Autodesk Fusion 360 part; units mm, degrees
sphere "SpherePrimitive2" add diameter 17 placed x (1, 0, 0) y (0, 0, -1) z (0, 1, 0) at (0, 0, 0) makes body 1
shell "Shell1" thickness 1 removed faces 0 bodies 1
ref_plane "WorkPlane1" through (0, 0, 3) normal (0, 0, 1) x (1, 0, 0)
split "Split1" by plane through (0, 0, 3) normal (0, 0, 1) bodies 1 makes body 2 at (-5.4981, 0.571, 6.4572)
delete_body "RemoveBody1" bodies 2
cylinder "CylinderPrimitive1" add diameter 17 height -22.5 placed x (1, 0, 0) y (0, 1, 0) z (0, 0, 1) at (0, 0, 0) separate body makes body 3
sphere "SpherePrimitive4" cut diameter 15 placed x (1, 0, 0) y (0, 0, -1) z (0, 1, 0) at (0, 0, 0) bodies 3
combine "Combine8" operation add target body 1 tool bodies 3
ref_plane "WorkPlane4" through (0, 8.5, -11.25) normal (0, 1, 0) x (1, 0, 0)
sketch "Sketch vis haut" plane through (0, 8.5, -4.25) normal (0, 1, 0) x (1, 0, 0)
  line L0 (0, 18.25) -> (0, 16.75)
  line L1 (-3, 18.25) -> (3, 18.25)
  line L2 (3, 18.25) -> (3, 15.25)
  line L3 (3, 15.25) -> (-3, 15.25)
  line L4 (-3, 15.25) -> (-3, 18.25)
  line L5 (0, 16.75) -> (0.1, 16.75)
  point P0 (0, 16.75)
  point P1 (0, 18.25)
  dimension "d72" = 1.5
  dimension "d73" = 3
  dimension "d74" = 6
extrude "Extrude4" add sketch "Sketch vis haut" along normal blind 6 and the other way blind 2 separate body makes body 4
hole "Hole1" at (0, 12.5, -19.5) direction (0, 0, -1) diameter 3 depth 3 tip angle 180 bodies 4
mirror "Mirror4" about plane through (0, 0, 0) normal (0, 1, 0) of bodies 4 makes body 5
combine "Combine9" operation add target body 1 tool bodies 4 5
sketch "Sketch13" plane through (0, 0, 3) normal (0, 0, 1) x (1, 0, 0)
  line L0 (9, 3.5) -> (-9, 3.5)
  line L1 (-9, 3.5) -> (-9, -3.5)
  line L2 (-9, -3.5) -> (9, -3.5)
  line L3 (9, -3.5) -> (9, 3.5)
  line L4 (9, 3.5) -> (-9, -3.5) construction
  line L5 (-9, 3.5) -> (9, -3.5) construction
  dimension "d54" = 7
  dimension "d55" = 18
extrude "Extrude5" cut sketch "Sketch13" against normal blind 10 bodies 1
Build history of the part. All positions in model axes, mm. A direction names the side the tool comes from. Give positions to 0.01 mm unless a question says otherwise; leave off trailing zeros. Loops run counter-clockwise (first coordinate to the right, second up) from the corner with the lowest first, then second, coordinate; pieces in that order, holes last. Notation, with made-up numbers: (-11, -40) -> (-2, -40) arc R17 cw to (-2, -14) -> close; hole circle Ø10 at (48, -8.5). An arc over 180 degrees is marked (long way). Answer in a Markdown table with one row per item.
Item 1: Tool access for faces 1 (the flat face through (-2, 2.4, -7)), 2 (the flat face through (-3, 11, -21)), 3 (the cylindrical face through (-8.49, 0.37, -11.09)), 4 (the flat face through (-3, -11, -21)), 5 (the flat face through (3, -11, -21)): list every direction of +Z, -Z, +X, -X, +Y, -Y with a clear straight run to the whole face (end or side of a thin tool).
Findings below:
| item | result |
|---|---|
| face 1 | +Z, +X, -X |
| face 2 | +Z, -Z, -X, +Y |
| face 3 | +Z |
| face 4 | +Z, -Z, -X, -Y |
| face 5 | +Z, -Z, +X, -Y |
Item 2: Slice it at A-A on y = -12.5. Write the cut outline in (x, z).
Findings below:
| item | result |
|---|---|
| outline | (-3, -22.5) -> (-1.5, -22.5) -> (-1.5, -19.5) -> (-3, -19.5) -> close; (1.5, -22.5) -> (3, -22.5) -> (3, -19.5) -> (1.5, -19.5) -> close |
Item 3: Slice it at D-D on y = 0. Write the cut outline in (x, z), plus the area to 3 significant figures.
Findings below:
| item | result |
|---|---|
| outline | (-8.5, -22.5) -> (8.5, -22.5) -> (8.5, -7) -> (2.69, -7) arc R7.5 cw to (-2.69, -7) -> (-8.5, -7) -> close |
| area | 262 mm² |
Item 4: Slice it at B-B on z = -6. Write the cut outline in (x, y), plus the area to 3 significant figures.
Findings below:
| item | result |
|---|---|
| outline | (-7.75, -3.5) arc R8.5 ccw to (7.75, -3.5) -> (2.83, -3.5) arc R4.5 cw to (-2.83, -3.5) -> close; (-7.75, 3.5) -> (-2.83, 3.5) arc R4.5 cw to (2.83, 3.5) -> (7.75, 3.5) arc R8.5 ccw to start |
| area | 104 mm² |
Item 5: Mould opens along Y. For faces 6 (the flat face through (0.6, 3.5, -6.8)), 7 (the flat face through (0, 0, -22.5)), 8 (the cylindrical face through (0, -14, -21)), 9 (the flat face through (0, -14.5, -21)) say: pulls with the +Y half, pulls with the -Y half, needs draft (parallel to the pull), parting line crosses it, or undercut.
Findings below:
| item | result |
|---|---|
| face 6 | undercut |
| face 7 | needs draft |
| face 8 | undercut |
| face 9 | pulls with the -Y half |
Item 6: Slice it at C-C on x = 0. Write the cut outline in (y, z), plus the area to 3 significant figures.
Findings below:
| item | result |
|---|---|
| outline | (-14.5, -22.5) -> (-14, -22.5) -> (-14, -19.5) -> (-14.5, -19.5) -> close; (-11, -22.5) -> (11, -22.5) -> (11, -19.5) -> (8.5, -19.5) -> (8.5, 0) arc R8.5 ccw to (7.95, 3) -> (6.87, 3) arc R7.5 cw to (3.5, -6.63) -> (3.5, -7) -> (2.69, -7) arc R7.5 cw to (-2.69, -7) -> (-3.5, -7) -> (-3.5, -6.63) arc R7.5 cw to (-6.87, 3) -> (-7.95, 3) arc R8.5 ccw to (-8.5, 0) -> (-8.5, -19.5) -> (-11, -19.5) -> close; (14, -22.5) -> (14.5, -22.5) -> (14.5, -19.5) -> (14, -19.5) -> close |
| area | 318 mm² |
Item 7: Flat gauge pins, fed straight in: P1, Ø3, axis at x = 0, y = -11, coming from the +Z side; P2, Ø10, axis at y = 8, z = -19, coming from the -X side; P3, Ø8, axis at x = -1.5, z = -3, coming from the -Y side; P4, Ø1.8, axis at x = 0, y = -12.5, coming from the -Z side. Where does each tip first touch, or does it go through?
Findings below:
| item | result |
|---|---|
| P1 | stops at z = -19.5 |
| P2 | stops at x = -7.95 |
| P3 | stops at y = -8.5 |
| P4 | passes through |
Item 8: Probe line 1 along Y through (x, z) = (0, -21); line 2 along X through (y, z) = (-12.5, -20.3); line 3 along Z through (x, y) = (5.75, 3). List the from-to ranges inside material, lowest first. Write a range as [from, to].
Findings below:
| item | result |
|---|---|
| line 1 | y = [-14.5, -14], [-11, 11], [14, 14.5] |
| line 2 | x = [-3, -1.5], [1.5, 3] |
| line 3 | z = [-22.5, -7] |
